Autodesk Inventor part; units mm, degrees
ref_plane "MSC_PT1" through (14.1, 0, 0) normal (1, 0, 0) x (0, 1, 0)
ref_plane "MSC_PT2" through (0, 0, 0) normal (-1, 0, 0) x (0, -1, 0)
ref_plane "MSC_PF1" through (0, 0, 0) normal (1, 0, 0) x (0, 1, 0)
sketch "Sketch1" plane through (0, 0, 0) normal (1, 0, 0) x (0, 1, 0)
  line L0 (10.5, 6.0622) -> (10.5, -6.0622)
  line L1 (10.5, -6.0622) -> (0, -12.1244)
  line L2 (0, -12.1244) -> (-10.5, -6.0622)
  line L3 (-10.5, -6.0622) -> (-10.5, 6.0622)
  line L4 (-10.5, 6.0622) -> (0, 12.1244)
  line L5 (0, 12.1244) -> (10.5, 6.0622)
  circle A0 centre (0, 0) radius 10.5 construction
  dimension "d0" = 21
extrude "Extrusion1" add sketch "Sketch1" along normal blind 14.1
sketch "Sketch2" plane through (14.1, 0, 0) normal (1, 0, 0) x (0, 1, 0)
  line L0 (-10.5, 6.0622) -> (0, 12.1244)
  line L1 (0, -12.1244) -> (-10.5, -6.0622)
  line L2 (-10.5, 6.0622) -> (10.5, -6.0622) construction
  line L3 (-10.5, -6.0622) -> (10.5, 6.0622) construction
  point P0 (0, 0)
hole "Hole1" at (14.1, 0, 0) direction (-1, 0, 0) diameter 11.835 end through all
chamfer "Chamfer1" distance 1 angle 45 2 edges at (14.1, 0, 5.9175) (0, 0, 5.9175)
sketch "Sketch3" plane through (0, 0, 0) normal (0, 1, 0) x (-1, 0, 0)
  line L0 (-17.0915, 0) -> (3.8489, 0)
  line L1 (-5.7048, 0) -> (0.8574, 0)
  line L2 (-14.1, 0) -> (-14.1, -12.1244)
  line L3 (-14.1, -12.1244) -> (0, -12.1244)
  line L4 (0, -12.1244) -> (0, 0)
  line L5 (-14.1, -6.0622) -> (-14.1, -12.1244)
  line L6 (0, -6.0622) -> (0, -12.1244)
  line L7 (0, -12.1244) -> (-14.1, -12.1244)
  line L8 (-14.1, -10.5) -> (-13.1622, -12.1244)
  line L9 (-14.1, -12.1244) -> (-14.1, -10.5)
  line L10 (-14.1, -12.1244) -> (-13.1622, -12.1244)
  line L11 (0, -10.5) -> (-0.9378, -12.1244)
  line L12 (-0.9378, -12.1244) -> (0, -12.1244)
  line L13 (0, -12.1244) -> (0, -10.5)
  dimension "d32" = 10.5
  dimension "d33" = 30
revolve "Revolution1" cut sketch "Sketch3" angle 360 about axis through (0, 0, 0) along (-1, 0, 0) contours L8 L3 L2 | L4 L3 L11
ref_plane "MSC_PT1" through (14.1, 0, 0) normal (1, 0, 0) x (0, 1, 0)
ref_plane "MSC_PT2" through (0, 0, 0) normal (-1, 0, 0) x (0, -1, 0)
ref_plane "MSC_PF1" through (0, 0, 0) normal (1, 0, 0) x (0, 1, 0)
equation "\"d0\" = Smax"
equation "\"d1\" = Mmax"
equation "\"d10\" = 0.5 * PTC"
equation "\"d32\" = 0.5 * Smax"
equation "\"NND\" = 14"
equation "\"Smax\" = 21"
equation "\"Mmax\" = 14.1"
equation "\"PTC\" = 2"
equation "\"THREADDIA\" = NND"
equation "\"TEMPLATE\" = 1.2345"
properties part number "ANSI B18.2.4.2M - M14x2" material "Steel, Mild"
Can you work these out from the model? Positions are in its coordinate system, mm. Give positions to 0.01 mm unless a question says otherwise; leave off trailing zeros. Loops run counter-clockwise (first coordinate to the right, second up) from the corner with the lowest first, then second, coordinate; pieces in that order, holes last. Notation, with made-up numbers: (86, 42.25) - (132, 42.25) arc R27 cw to (132, 58.25) - close; hole circle Ø11 at (74.25, 1). An arc over 180 degrees is marked (long way). Return JSON: item names as keys, results as strings.
1. I'm going to push flat-ended pins straight in: pin 1 Ø1 at (x, z) = (8.5, -9) entering from +Y; pin 2 Ø2 at (x, y) = (7, -1.5) entering from +Z. Where does each tip first touch, or does it pass through?
Output values:
{"pin 1": "stops at y = 6.28", "pin 2": "stops at z = 11.84"}
2. If I drill on line 1 (Y direction, x = 5.25, z = 0); line 2 (Z direction, x = 7.25, y = 3.5); line 3 (Y direction, x = 8, z = 3.75), over which ranges is the centre line in solid material (lowest first)?
Output values:
{"line 1": "y = -10.5 to -5.92, 5.92 to 10.5", "line 2": "z = -10.1 to -4.77, 4.77 to 10.1", "line 3": "y = -10.5 to -4.58, 4.58 to 10.5"}
3. We'd pull the mould along Z, two halves only. Please class faces 1 (the face through (0, 2, -7)), 2 (the face through (6.965, -5.867, 0.77)), 3 (the face through (0.161, 0.237, 10.776)), 4 (the face through (6.951, -5.176, -9.136)): +Z half, -Z half, draft (parallel to the pull), parting line (faces both ways), or undercut.
Output values:
{"face 1": "draft", "face 2": "undercut", "face 3": "+Z half", "face 4": "-Z half"}
4. I want a section at A-A on x = 10.5. Please give me the cut outline in (y, z) (1 decimal).
Output values:
{"outline": "(-10.5, -6.1) - (0, -12.1) - (10.5, -6.1) - (10.5, 6.1) - (0, 12.1) - (-10.5, 6.1) - close; hole circle Ø11.8 at (0, 0)"}
